```python
from build123d import *

# Parameters (mm, degrees)
SKETCH1_W               = 100
SKETCH1_H               = 100
BOSS_EXTRUDE1_DEPTH     = 68.7
SKETCH2_R               = 40
CUT_EXTRUDE1_DEPTH      = 10
SKETCH3_R               = 28.5
CUT_EXTRUDE2_DEPTH      = 6.1
CUT_EXTRUDE3_DEPTH      = 89.129223303
CUT_EXTRUDE3_DEPTH_BACK = 15.01
SKETCH4_W               = 20.11
SKETCH4_H               = 55.01
SKETCH5_W               = 20.11
SKETCH5_H               = 40.11
CUT_EXTRUDE4_DEPTH      = 27.51
CUT_EXTRUDE5_REACH      = 133.224
SKETCH7_R               = 2.775
CUT_EXTRUDE6_DEPTH      = 3.2
CUT_EXTRUDE7_DEPTH      = 5
SKETCH9_W               = 120
SKETCH9_H               = 120
BOSS_EXTRUDE2_DEPTH     = 5
FILLET2_R               = 3


with BuildPart() as part:
    # Sketch1 → Boss-Extrude1 (new body)
    with BuildSketch(Plane(origin=(0, 0, 0), x_dir=(1, 0, 0), z_dir=(0, 1, 0))):
        Rectangle(SKETCH1_W, SKETCH1_H)
    extrude(amount=BOSS_EXTRUDE1_DEPTH)

    # Sketch2 → Cut-Extrude1 (cut)
    with BuildSketch(Plane(origin=(0, 68.7, 0), x_dir=(1, 0, 0), z_dir=(0, 1, 0))):
        with Locations(Location((0, 0, 0), (0, 0, 270))):
            Circle(SKETCH2_R)
    extrude(amount=-CUT_EXTRUDE1_DEPTH, mode=Mode.SUBTRACT)

    # Sketch3 → Cut-Extrude2 (cut)
    with BuildSketch(Plane(origin=(0, 58.7, 0), x_dir=(1, 0, 0), z_dir=(0, 1, 0))):
        with Locations(Location((0, 0, 0), (0, 0, 270))):
            Circle(SKETCH3_R)
    extrude(amount=-CUT_EXTRUDE2_DEPTH, mode=Mode.SUBTRACT)

    # Sketch4 → Cut-Extrude3 (cut, two sides: drawn at the far end of the back side and taken through both)
    with BuildSketch(Plane(origin=(0, 52.6, 0), x_dir=(1, 0, 0), z_dir=(0, 1, 0)).offset(-CUT_EXTRUDE3_DEPTH_BACK)):
        with Locations((0, -10.005)):
            Rectangle(SKETCH4_W, SKETCH4_H)
    extrude(amount=CUT_EXTRUDE3_DEPTH + CUT_EXTRUDE3_DEPTH_BACK, mode=Mode.SUBTRACT)

    # Sketch5 → Cut-Extrude4 (cut)
    with BuildSketch(Plane(origin=(0, 37.59, 0), x_dir=(1, 0, 0), z_dir=(0, 1, 0))):
        with Locations((0, -10.055)):
            Rectangle(SKETCH5_W, SKETCH5_H)
    extrude(amount=-CUT_EXTRUDE4_DEPTH, mode=Mode.SUBTRACT)

    # Sketch6 → Cut-Extrude5 (cut, up to next)
    with BuildSketch(Plane(origin=(0, 0, -50), x_dir=(-1, 0, 0), z_dir=(0, 0, -1)), mode=Mode.PRIVATE) as cut_extrude5_sk1:
        with BuildLine():
            Line((-3.5, 13.08), (3.5, 13.08))
            Line((3.5, 13.08), (3.5, 17.58))
            ThreePointArc((3.5, 17.58), (0, 21.08), (-3.5, 17.58))
            Line((-3.5, 17.58), (-3.5, 13.08))
        make_face()
    cut_extrude5_tool1 = extrude(cut_extrude5_sk1.sketch, amount=-CUT_EXTRUDE5_REACH, mode=Mode.PRIVATE) & part.part
    add(cut_extrude5_tool1.solids().sort_by_distance((0, 16.746539, -50))[0], mode=Mode.SUBTRACT)

    # Sketch7 → Cut-Extrude6 (cut)
    with BuildSketch(Plane(origin=(0, 37.59, 0), x_dir=(1, 0, 0), z_dir=(0, 1, 0))):
        with Locations(Location((5.055, -34.01, 0), (0, 0, 270))):
            Circle(SKETCH7_R)
        with Locations(Location((-5.055, -34.01, 0), (0, 0, 270))):
            Circle(SKETCH7_R)
        with Locations(Location((-5.055, 14, 0), (0, 0, 270))):
            Circle(SKETCH7_R)
        with Locations(Location((5.055, 14, 0), (0, 0, 270))):
            Circle(SKETCH7_R)
    extrude(amount=-CUT_EXTRUDE6_DEPTH, mode=Mode.SUBTRACT)

    # Sketch8 → Cut-Extrude7 (cut)
    with BuildSketch(Plane.XY.offset(-10)):
        with BuildLine():
            Line((-3.5, 13.08), (3.5, 13.08))
            Line((3.5, 13.08), (3.5, 31.08))
            ThreePointArc((3.5, 31.08), (0, 34.58), (-3.5, 31.08))
            Line((-3.5, 31.08), (-3.5, 13.08))
        make_face()
    extrude(amount=-CUT_EXTRUDE7_DEPTH, mode=Mode.SUBTRACT)

    # Sketch9 → Boss-Extrude2 (add)
    with BuildSketch(Plane.XZ):
        Rectangle(SKETCH9_W, SKETCH9_H)
    extrude(amount=-BOSS_EXTRUDE2_DEPTH)

    # Fillet2
    fillet2_edges = [part.edges().sort_by_distance(p)[0] for p in [
        (-50, 5, 0),
        (50, 5, 0),
        (0, 5, 50),
        (60, 5, 0),
        (0, 5, -60),
        (-60, 5, 0),
        (0, 5, 60),
        (0, 5, -50),
        (0, 68.7, -50),
        (-50, 68.7, 0),
        (0, 68.7, 50),
        (-50, 36.85, 50),
        (-50, 36.85, -50),
        (50, 36.85, -50),
        (50, 36.85, 50),
        (50, 68.7, 0),
    ]]
    fillet(fillet2_edges, radius=FILLET2_R)


solid = part.part
```
Here's how the part is built. I have some questions about the finished solid (model axes, mm). A direction names the side the tool comes from. Coordinates: 2 decimals unless noted, no trailing zeros. Loops run counter-clockwise (first coordinate to the right, second up) from the corner with the lowest first, then second, coordinate; pieces in that order, holes last. Notation, with made-up numbers: (26, 8) - (67, 8) arc R19 ccw to (67, 34) - close; hole circle Ø5 at (57.25, -20.75). An arc over 180 degrees is marked (long way). Return JSON: item names as keys, results as strings. Group by question number.
Item 1: If we section it at B-B on y = 39.5: Write out the boundary of the cut face in (x, z) (3 decimals), and give its area (3 significant figures).
Item 2: If we section it at C-C on z = -24.5: Write out the boundary of the cut face in (x, y).
Item 3: Will these pins go through, and if not, where does the flat tip stop? P1, Ø7.5, axis at x = -1.5, y = 26.5, coming from the +Z side; P2, Ø10, axis at x = 39.5, y = 51.5, coming from the -Z side; P3, Ø3.5, axis at x = -5.055, z = -14, coming from the +Y side.
Item 4: On a 3-axis mill with a long thin cutter (end or side, diameter ignored), from which of +Z, -Z, +X, -X, +Y, -Y can I reach the whole of each face in a straight line? I mean faces 4 (the face through (49.1, 37.25, -49.14)), 5 (the face through (-49.1, 37.25, -49.14)), 6 (the face through (10.055, 34, 10)). Say none if no direction works.
Item 5: If we section it at D-D on z = 0: Write out the boundary of the cut face in (x, y) (3 decimals).
Item 6: We'd pull the mould along X, two halves only. Please class faces 1 (the face through (-42, 68.7, -1)), 2 (the face through (-50, 36, 1)), 3 (the face through (-12, 52.6, -1)): +X half, -X half, draft (parallel to the pull), parting line (faces both ways), or undercut.
Item 7: I need wall thicknesses on line 1 (X direction, y = 36, z = -14); line 2 (X direction, y = 65.25, z = 0); line 3 (X direction, y = 43.5, z = 35.5) (3 decimals). Which ranges of each line are inside material? Lowest first, please. Write a range as from..to.
Calculated:
{
 "1": {"outline": "(-50, -47) arc R3 ccw to (-47, -50) - (47, -50) arc R3 ccw to (50, -47) - (50, 47) arc R3 ccw to (47, 50) - (-47, 50) arc R3 ccw to (-50, 47) - close; hole (-10.055, -17.5) - (10.055, -17.5) - (10.055, 37.51) - (-10.055, 37.51) - close", "area": "8,890 mm^2"},
 "2": {"outline": "(-60, 0) - (60, 0) - (60, 2) arc R3 ccw to (57, 5) - (53, 5) arc R3 cw to (50, 8) - (50, 65.7) arc R3 ccw to (47, 68.7) - (31.62, 68.7) - (31.62, 58.7) - (14.56, 58.7) - (14.56, 52.6) - (-14.56, 52.6) - (-14.56, 58.7) - (-31.62, 58.7) - (-31.62, 68.7) - (-47, 68.7) arc R3 ccw to (-50, 65.7) - (-50, 8) arc R3 cw to (-53, 5) - (-57, 5) arc R3 ccw to (-60, 2) - close; hole (-3.5, 13.08) - (3.5, 13.08) - (3.5, 17.58) arc R3.5 ccw to (-3.5, 17.58) - close"},
 "3": {"P1": "stops at z = 50", "P2": "stops at z = -50", "P3": "stops at y = 34.39"},
 "4": {"face 4": "-Z, +X, +Y", "face 5": "-Z, -X, +Y", "face 6": "+Y"},
 "5": {"outline": "(-60, 0) - (60, 0) - (60, 2) arc R3 ccw to (57, 5) - (53, 5) arc R3 cw to (50, 8) - (50, 65.7) arc R3 ccw to (47, 68.7) - (40, 68.7) - (40, 58.7) - (28.5, 58.7) - (28.5, 52.6) - (10.055, 52.6) - (10.055, 10.08) - (-10.055, 10.08) - (-10.055, 52.6) - (-28.5, 52.6) - (-28.5, 58.7) - (-40, 58.7) - (-40, 68.7) - (-47, 68.7) arc R3 ccw to (-50, 65.7) - (-50, 8) arc R3 cw to (-53, 5) - (-57, 5) arc R3 ccw to (-60, 2) - close"},
 "6": {"face 1": "draft", "face 2": "-X half", "face 3": "undercut"},
 "7": {"line 1": "x = -50..-7.83, -2.28..2.28, 7.83..50", "line 2": "x = -50..-40, 40..50", "line 3": "x = -50..-10.055, 10.055..50"}
}
